Geometry: see drawing. Coordinates: mm, zero at the bounding-box minimum. Coordinates: 2 decimals unless noted, no trailing zeros. Order: outer loops, then holes, each group sorted by start corner. A loop starts at its lowest first (then second) coordinate and runs counter-clockwise, first axis right, second up.
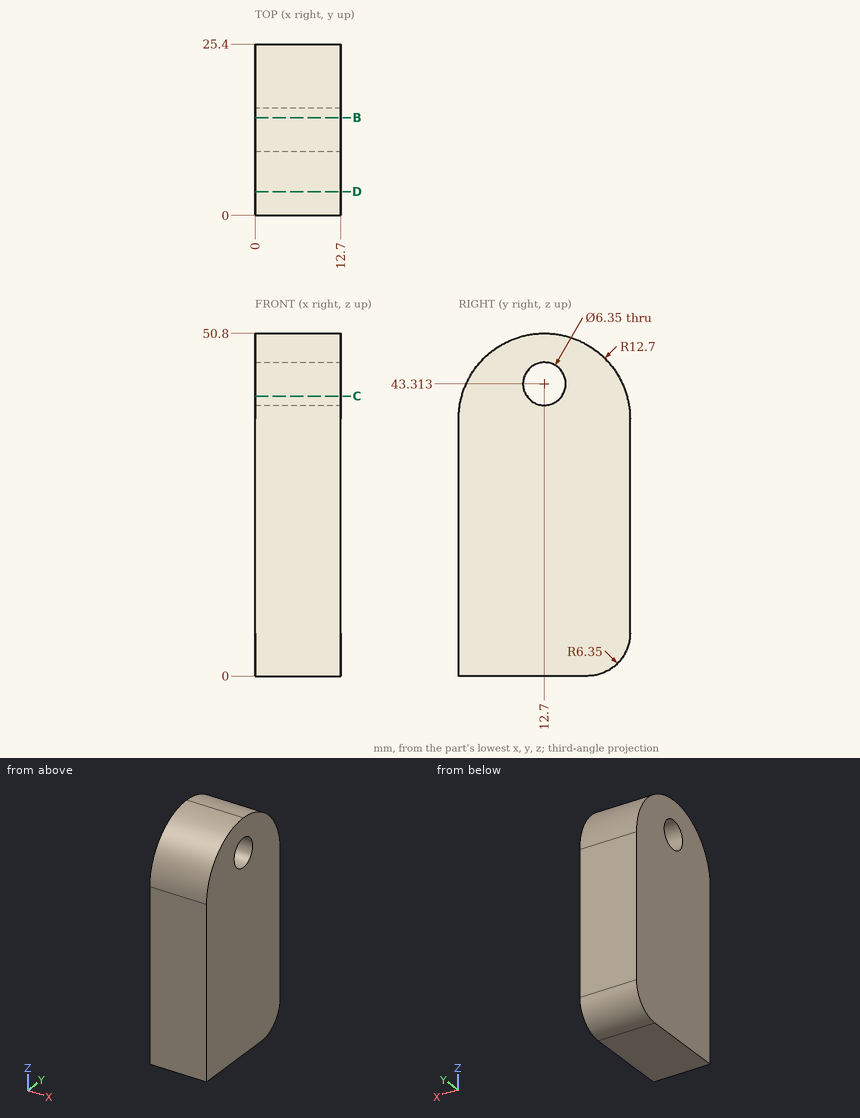
Item 1: Cut plane C-C on z = 41.5. Return loops of the section in (x, y), then the cut area to 3 significant figures.
Response values:
outline: (0, 0.46) - (12.7, 0.46) - (12.7, 10.09) - (0, 10.09) - close; (0, 15.31) - (12.7, 15.31) - (12.7, 24.94) - (0, 24.94) - close
area: 245 mm2
Item 2: Pin query (flat end, axial travel): pin 1 Ø3 at (x, y) = (4, 11) entering from +Z; pin 2 Ø1 at (x, z) = (5.5, 45.5) entering from -Y. Return the tip coordinate at first contact, or that it passes through.
Response values:
pin 1: stops at z = 50.8
pin 2: stops at y = 2.04
Item 3: Cut plane D-D on y = 3.5. Return loops of the section in (x, z) (1 decimal).
Response values:
outline: (0, 0) - (12.7, 0) - (12.7, 46.9) - (0, 46.9) - close
Item 4: Cut plane B-B on y = 14.5. Return loops of the section in (x, z), then the cut area to 3 significant figures.
Response values:
outline: (0, 0) - (12.7, 0) - (12.7, 40.7) - (0, 40.7) - close; (0, 45.93) - (12.7, 45.93) - (12.7, 50.67) - (0, 50.67) - close
area: 577 mm2
Item 5: Ray query, probe 1 along Z at (x, y) = (8, 12.7); probe 2 along Z at (x, y) = (3.5, 13.5) (1 decimal); probe 3 along Y at (x, z) = (2, 40.5). Return the intervals inside material, ascending.
Response values:
probe 1: z = 0 to 40.14, 46.49 to 50.8
probe 2: z = 0 to 40.2, 46.4 to 50.8
probe 3: y = 0.23 to 11.23, 14.17 to 25.17
